Autodesk Inventor part; units mm, degrees
ref_plane "YZ Plane" through (0, 0, 0) normal (1, 0, 0) x (0, 1, 0)
ref_plane "XZ Plane" through (0, 0, 0) normal (0, 1, 0) x (-1, 0, 0)
ref_plane "XY Plane" through (0, 0, 0) normal (0, 0, 1) x (1, 0, 0)
sketch "Sketch1" plane through (0, 0, 0) normal (0, 0, 1) x (1, 0, 0)
  line L0 (0, 0) -> (25.4, 0)
  line L1 (25.4, 0) -> (25.4, 50.8)
  line L2 (25.4, 50.8) -> (0, 50.8)
  line L3 (0, 50.8) -> (0, 0)
  line L4 (22.8651, 48.2651) -> (22.8651, 2.5349)
  line L5 (22.8651, 2.5349) -> (2.5349, 2.5349)
  line L6 (2.5349, 2.5349) -> (2.5349, 48.2651)
  line L7 (2.5349, 48.2651) -> (22.8651, 48.2651)
  dimension "d0" = 25.4
  dimension "d1" = 50.8
  dimension "d2" = 2.5349
extrude "Extrusion1" add sketch "Sketch1" along normal blind 444.5
sketch "Sketch2" plane through (0, 50.8, 0) normal (0, 1, 0) x (1, 0, 0)
  line L0 (0, 0) -> (12.7, 0)
  line L1 (25.4, 0) -> (0, 0)
  line L2 (0, 0) -> (0, -444.5)
  line L3 (12.7, 0) -> (12.7, -25.4)
  circle A0 centre (12.7, -25.4) radius 1.9939
  line L4 (12.7, -25.4) -> (12.7, -50.8)
  circle A1 centre (12.7, -50.8) radius 1.9939
  line L5 (12.7, -50.8) -> (12.7, -76.2)
  circle A2 centre (12.7, -76.2) radius 1.9939
  line L6 (12.7, -25.4) -> (12.7, -50.8)
  circle A3 centre (12.7, -50.8) radius 1.9939
  line L7 (12.7, -50.8) -> (12.7, -76.2)
  circle A4 centre (12.7, -76.2) radius 1.9939
  line L8 (12.7, -76.2) -> (12.7, -101.6)
  circle A5 centre (12.7, -101.6) radius 1.9939
  line L9 (12.7, -50.8) -> (12.7, -76.2)
  circle A6 centre (12.7, -76.2) radius 1.9939
  line L10 (12.7, -76.2) -> (12.7, -101.6)
  circle A7 centre (12.7, -101.6) radius 1.9939
  line L11 (12.7, -101.6) -> (12.7, -127)
  circle A8 centre (12.7, -127) radius 1.9939
  line L12 (12.7, -76.2) -> (12.7, -101.6)
  circle A9 centre (12.7, -101.6) radius 1.9939
  line L13 (12.7, -101.6) -> (12.7, -127)
  circle A10 centre (12.7, -127) radius 1.9939
  line L14 (12.7, -127) -> (12.7, -152.4)
  circle A11 centre (12.7, -152.4) radius 1.9939
  line L15 (12.7, -101.6) -> (12.7, -127)
  circle A12 centre (12.7, -127) radius 1.9939
  line L16 (12.7, -127) -> (12.7, -152.4)
  circle A13 centre (12.7, -152.4) radius 1.9939
  line L17 (12.7, -152.4) -> (12.7, -177.8)
  circle A14 centre (12.7, -177.8) radius 1.9939
  line L18 (12.7, -127) -> (12.7, -152.4)
  circle A15 centre (12.7, -152.4) radius 1.9939
  line L19 (12.7, -152.4) -> (12.7, -177.8)
  circle A16 centre (12.7, -177.8) radius 1.9939
  line L20 (12.7, -177.8) -> (12.7, -203.2)
  circle A17 centre (12.7, -203.2) radius 1.9939
  line L21 (12.7, -152.4) -> (12.7, -177.8)
  circle A18 centre (12.7, -177.8) radius 1.9939
  line L22 (12.7, -177.8) -> (12.7, -203.2)
  circle A19 centre (12.7, -203.2) radius 1.9939
  line L23 (12.7, -203.2) -> (12.7, -228.6)
  circle A20 centre (12.7, -228.6) radius 1.9939
  line L24 (12.7, -177.8) -> (12.7, -203.2)
  circle A21 centre (12.7, -203.2) radius 1.9939
  line L25 (12.7, -203.2) -> (12.7, -228.6)
  circle A22 centre (12.7, -228.6) radius 1.9939
  line L26 (12.7, -228.6) -> (12.7, -254)
  circle A23 centre (12.7, -254) radius 1.9939
  line L27 (12.7, -203.2) -> (12.7, -228.6)
  circle A24 centre (12.7, -228.6) radius 1.9939
  line L28 (12.7, -228.6) -> (12.7, -254)
  circle A25 centre (12.7, -254) radius 1.9939
  line L29 (12.7, -254) -> (12.7, -279.4)
  circle A26 centre (12.7, -279.4) radius 1.9939
  line L30 (12.7, -228.6) -> (12.7, -254)
  circle A27 centre (12.7, -254) radius 1.9939
  line L31 (12.7, -254) -> (12.7, -279.4)
  circle A28 centre (12.7, -279.4) radius 1.9939
  line L32 (12.7, -279.4) -> (12.7, -304.8)
  circle A29 centre (12.7, -304.8) radius 1.9939
  line L33 (12.7, -254) -> (12.7, -279.4)
  circle A30 centre (12.7, -279.4) radius 1.9939
  line L34 (12.7, -279.4) -> (12.7, -304.8)
  circle A31 centre (12.7, -304.8) radius 1.9939
  line L35 (12.7, -304.8) -> (12.7, -330.2)
  circle A32 centre (12.7, -330.2) radius 1.9939
  line L36 (12.7, -279.4) -> (12.7, -304.8)
  circle A33 centre (12.7, -304.8) radius 1.9939
  line L37 (12.7, -304.8) -> (12.7, -330.2)
  circle A34 centre (12.7, -330.2) radius 1.9939
  line L38 (12.7, -330.2) -> (12.7, -355.6)
  circle A35 centre (12.7, -355.6) radius 1.9939
  line L39 (12.7, -304.8) -> (12.7, -330.2)
  circle A36 centre (12.7, -330.2) radius 1.9939
  line L40 (12.7, -330.2) -> (12.7, -355.6)
  circle A37 centre (12.7, -355.6) radius 1.9939
  line L41 (12.7, -355.6) -> (12.7, -381)
  circle A38 centre (12.7, -381) radius 1.9939
  line L42 (12.7, -330.2) -> (12.7, -355.6)
  circle A39 centre (12.7, -355.6) radius 1.9939
  line L43 (12.7, -355.6) -> (12.7, -381)
  circle A40 centre (12.7, -381) radius 1.9939
  line L44 (12.7, -381) -> (12.7, -406.4)
  circle A41 centre (12.7, -406.4) radius 1.9939
  line L45 (12.7, -355.6) -> (12.7, -381)
  circle A42 centre (12.7, -381) radius 1.9939
  line L46 (12.7, -381) -> (12.7, -406.4)
  circle A43 centre (12.7, -406.4) radius 1.9939
  line L47 (12.7, -406.4) -> (12.7, -431.8)
  circle A44 centre (12.7, -431.8) radius 1.9939
  dimension "d5" = 25.4
  dimension "d6" = 3.9878
  dimension "d7" = 25.4
  dimension "d8" = 3.9878
  dimension "d9" = 25.4
  dimension "d10" = 3.9878
  dimension "d29" = 25.4
extrude "Extrusion2" cut sketch "Sketch2" against normal blind 444.5
properties part number "RobotBaseSide"
For this review, take the finished solid that the model builds, in its own axes (mm). A direction names the side the tool comes from. Coordinates: 2 decimals unless noted, no trailing zeros. Order: outer loops, then holes, each group sorted by start corner. A loop starts at its lowest first (then second) coordinate and runs counter-clockwise, first axis right, second up. Notation, with made-up numbers: (-30.75, 71) -> (13.25, 71) arc R20 ccw to (13.25, 87) -> close; hole circle Ø6 at (72.25, 33). An arc over 180 degrees is marked (long way). Answer as CSV lines item,"result".
Q1. For faces 1 (the face through (13, 0, 219)), 2 (the face through (22.865, 26, 219)), list the 3-axis set-ups (+Z, -Z, +X, -X, +Y, -Y) from which the entire face can be reached by the end or side of a thin tool; tool diameter is ignored.
Model answer:
face 1,"+Z, -Z, +X, -X, -Y"
face 2,"+Z, -Z"
Q2. We need section A-A (y = 32.5). State the section outline as (x, z) points.
Model answer:
outline,"(0, 0) -> (2.53, 0) -> (2.53, 444.5) -> (0, 444.5) -> close; (22.87, 0) -> (25.4, 0) -> (25.4, 444.5) -> (22.87, 444.5) -> close"
Q3. Draft analysis for pull direction Y (two halves, no side actions). For faces 3 (the face through (25.4, 25, 219)), 4 (the face through (13, 2.535, 219)), 5 (the face through (13, 50.8, 219)), state which applies: released by +Y, released by -Y, zero draft, split by the parting line, or undercut.
Model answer:
face 3,"zero draft"
face 4,"undercut"
face 5,"released by +Y"
Q4. We need section B-B (z = 66.5). State the section outline as (x, y) points, plus the area to 3 significant figures.
Model answer:
outline,"(0, 0) -> (25.4, 0) -> (25.4, 50.8) -> (0, 50.8) -> close; hole (2.53, 2.53) -> (22.87, 2.53) -> (22.87, 48.27) -> (2.53, 48.27) -> close"
area,"361 mm2"
Q5. Clearance check with a flat-ended pin moving along its axis: pin 1 Ø3 at (x, z) = (12.7, 177.8) entering from -Y. State where the tip first meets the part, or that it passes through.
Model answer:
pin 1,"passes through"
Q6. Wall thickness on line 1 along Y through (x, z) = (17.5, 318); line 2 along X through (y, z) = (48, 228); line 3 along X through (y, z) = (50.15, 304.8): over which ranges is each line inside the solid? List them lowest first. Write a range as [from, to].
Model answer:
line 1,"y = [0, 2.53], [48.27, 50.8]"
line 2,"x = [0, 2.53], [22.87, 25.4]"
line 3,"x = [0, 10.71], [14.69, 25.4]"
